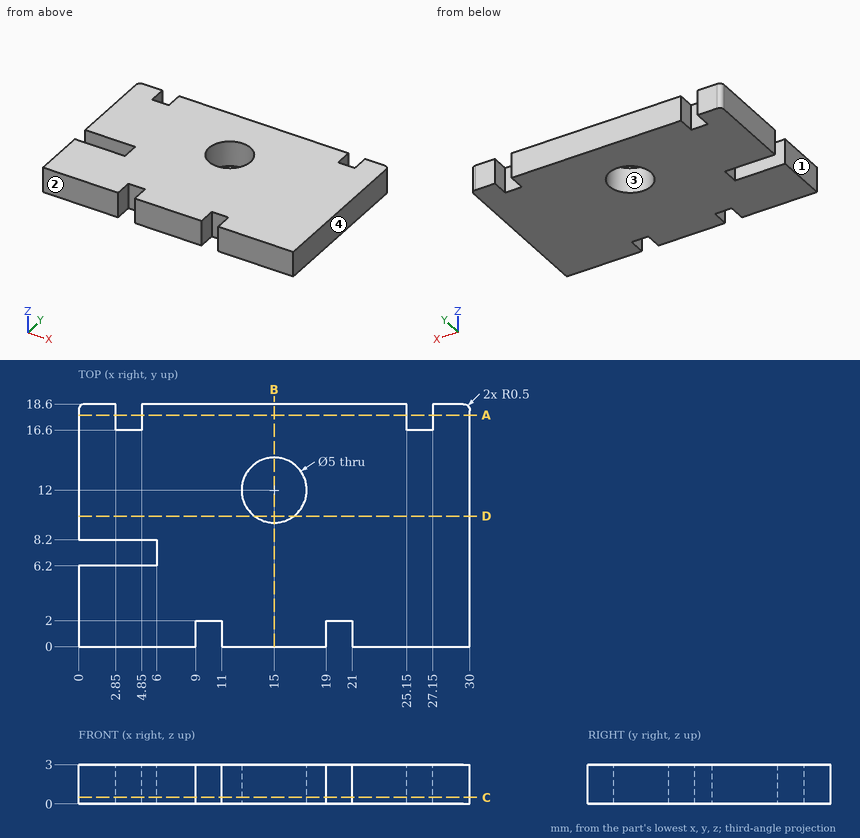
Check sheet for the drawn part. Datum: minimum x, y, z corner. Units: mm. Give positions to 0.01 mm unless a question says otherwise; leave off trailing zeros. Order: outer loops, then holes, each group sorted by start corner. A loop starts at its lowest first (then second) coordinate and runs counter-clockwise, first axis right, second up. Notation, with made-up numbers: (-31, 31) - (0, 31) arc R4 ccw to (0, 35) - close; hole circle Ø3 at (88, 19.25). An arc over 180 degrees is marked (long way). Answer in a Markdown table with one row per item. Add a question column.
Q1. Gauge pin test, flat ends, axial feed: pin 1 (0.6 mm diameter, centred on x = 10, z = 2, fed in from -Y); pin 2 (0.6 mm diameter, centred on y = 7, z = 1.5, fed in from -X); pin 3 (1.5 mm diameter, centred on x = 14, z = 2.5, fed in from -Y); pin 4 (0.6 mm diameter, centred on x = 26, z = 1, fed in from +Y). Record the tip position at first contact, or that the pin passes through.
Q2. Mould release check, pull along X, two halves, no side actions. Record for the marked faces 1, 2, 3 and 4: pulls with the +X half, pulls with the -X half, needs draft (parallel to the pull), parting line crosses it, or undercut.
Q3. Material ranges on probe 1 along Y at (x, z) = (5.75, 2.5); probe 2 along Y at (x, z) = (15, 2.35); probe 3 along X at (y, z) = (14.25, 0.4), recorded low to high. Write a range as from..to.
Q4. Cross-section at C-C, the plane z = 0.5. Enter the section's corners in (x, y), then the cut area to 3 significant figures.
Q5. Cross-section at A-A, the plane y = 17.75. Enter the section's corners in (x, z).
Q6. Cross-section at D-D, the plane y = 10. Enter the section's corners in (x, z), then the cut area to 3 significant figures.
Q7. Cross-section at B-B, the plane x = 15. Enter the section's corners in (y, z), then the cut area to 3 significant figures.
Check values:
| question | item | result |
|---|---|---|
| 1 | pin 1 | stops at y = 2 |
| 1 | pin 2 | stops at x = 6 |
| 1 | pin 3 | stops at y = 0 |
| 1 | pin 4 | stops at y = 16.6 |
| 2 | face 1 | pulls with the -X half |
| 2 | face 2 | needs draft |
| 2 | face 3 | undercut |
| 2 | face 4 | pulls with the +X half |
| 3 | probe 1 | y = 0..6.2, 8.2..18.6 |
| 3 | probe 2 | y = 0..9.5, 14.5..18.6 |
| 3 | probe 3 | x = 0..13.91, 16.09..30 |
| 4 | outline | (0, 0) - (9, 0) - (9, 2) - (11, 2) - (11, 0) - (19, 0) - (19, 2) - (21, 2) - (21, 0) - (30, 0) - (30, 18.1) arc R0.5 ccw to (29.5, 18.6) - (27.15, 18.6) - (27.15, 16.6) - (25.15, 16.6) - (25.15, 18.6) - (4.85, 18.6) - (4.85, 16.6) - (2.85, 16.6) - (2.85, 18.6) - (0.5, 18.6) arc R0.5 ccw to (0, 18.1) - (0, 8.2) - (6, 8.2) - (6, 6.2) - (0, 6.2) - close; hole circle Ø5 at (15, 12) |
| 4 | area | 510 mm^2 |
| 5 | outline | (0, 0) - (2.85, 0) - (2.85, 3) - (0, 3) - close; (4.85, 0) - (25.15, 0) - (25.15, 3) - (4.85, 3) - close; (27.15, 0) - (30, 0) - (30, 3) - (27.15, 3) - close |
| 6 | outline | (0, 0) - (13.5, 0) - (13.5, 3) - (0, 3) - close; (16.5, 0) - (30, 0) - (30, 3) - (16.5, 3) - close |
| 6 | area | 81.0 mm^2 |
| 7 | outline | (0, 0) - (9.5, 0) - (9.5, 3) - (0, 3) - close; (14.5, 0) - (18.6, 0) - (18.6, 3) - (14.5, 3) - close |
| 7 | area | 40.8 mm^2 |
